Here's how the part is built. I have some questions about the finished solid (model axes, mm). A direction names the side the tool comes from. Give positions to 0.01 mm unless a question says otherwise; leave off trailing zeros. Loops run counter-clockwise (first coordinate to the right, second up) from the corner with the lowest first, then second, coordinate; pieces in that order, holes last. Notation, with made-up numbers: (-11, 54.5) - (-3, 54.5) arc R28 cw to (-3, 75.5) - close; hole circle Ø10 at (-32, 40.5). An arc over 180 degrees is marked (long way). Return JSON: item names as keys, results as strings. Group by question number.
(1) On a 3-axis mill with a long thin cutter (end or side, diameter ignored), from which of +Z, -Z, +X, -X, +Y, -Y can I reach the whole of each face in a straight line? I mean faces 5 (the flat face through (75, 0, 7)), 6 (the cylindrical face through (-65, 0, 7)). Say none if no direction works.
(2) For P1, Ø8, axis at y = -22.5, z = 2.5, coming from the -X side, with a flat end and sliding along its axis, tell me the tip position at first contact or that it passes through.
(3) I need wall thicknesses on probe 1 along Y at (x, z) = (-37.5, 1); probe 2 along X at (y, z) = (20, 3.25); probe 3 along X at (y, z) = (0, 4). Which ranges of each line are inside material? Lowest first, please. Write a range as [from, to].
(4) If we section it at A-A (y = 0): Please give me the cut outline in (x, z).
(5) If we section it at C-C (z = 7.5): Please give me the cut outline in (x, y).
(6) If we section it at B-B (x = 0): Please give me the cut outline in (y, z).
(7) If we mould it in two halves opening along Y, with no side actions, what happens to faces 1 (the flat face through (65, 30, 7)), 2 (the flat face through (10, 15, 7)), 3 (the flat face through (1, -40, 7)), 4 (the flat face through (-75, 0, 7))? For each: released by +Y, released by -Y, zero draft, split by the parting line, or undercut.
```python
from build123d import *

# Parameters (mm, degrees)
BOSS_EXTRUDE1_DEPTH = 15


with BuildPart() as part:
    # Sketch1 → Boss-Extrude1 (new body)
    with BuildSketch(Plane.XY):
        Polygon((-75, 20), (-55, 40), (55, 40), (75, 20), (75, -20), (55, -40), (-55, -40), (-75, -20), align=None)
        with BuildLine():
            Line((-10, 10), (-10, 20))
            ThreePointArc((-10, 20), (0, 30), (10, 20))
            Line((10, 20), (10, 10))
            Line((10, 10), (55, 10))
            ThreePointArc((55, 10), (65, 0), (55, -10))
            Line((55, -10), (10, -10))
            Line((10, -10), (10, -20))
            ThreePointArc((10, -20), (0, -30), (-10, -20))
            Line((-10, -20), (-10, -10))
            Line((-10, -10), (-55, -10))
            ThreePointArc((-55, -10), (-65, 0), (-55, 10))
            Line((-55, 10), (-10, 10))
        make_face(mode=Mode.SUBTRACT)
    extrude(amount=BOSS_EXTRUDE1_DEPTH)


solid = part.part
```
Values:
{
 "1": {"face 5": "+Z, -Z, +X, +Y, -Y", "face 6": "+Z, -Z"},
 "2": {"P1": "x = -75"},
 "3": {"probe 1": "[-40, -10], [10, 40]", "probe 2": "[-75, -10], [10, 75]", "probe 3": "[-75, -65], [65, 75]"},
 "4": {"outline": "(-75, 0) - (-65, 0) - (-65, 15) - (-75, 15) - close; (65, 0) - (75, 0) - (75, 15) - (65, 15) - close"},
 "5": {"outline": "(-75, -20) - (-55, -40) - (55, -40) - (75, -20) - (75, 20) - (55, 40) - (-55, 40) - (-75, 20) - close; hole (-55, -10) - (-10, -10) - (-10, -20) arc R10 ccw to (10, -20) - (10, -10) - (55, -10) arc R10 ccw to (55, 10) - (10, 10) - (10, 20) arc R10 ccw to (-10, 20) - (-10, 10) - (-55, 10) arc R10 ccw to start"},
 "6": {"outline": "(-40, 0) - (-30, 0) - (-30, 15) - (-40, 15) - close; (30, 0) - (40, 0) - (40, 15) - (30, 15) - close"},
 "7": {"face 1": "released by +Y", "face 2": "undercut", "face 3": "released by -Y", "face 4": "zero draft"}
}
